Read the model definition and answer for the solid it produces. Units are mm, in the model's axes. A direction names the side the tool comes from. Coordinates: 2 decimals unless noted, no trailing zeros. Write each loop counter-clockwise with the first axis right and the second up, starting at its lowest first coordinate (ties: lowest second). Pieces come first, ordered by that corner, then holes. Notation, with made-up numbers: (5, 75) -> (21, 75) arc R18 cw to (21, 102) -> close; hole circle Ø1 at (-6.75, -40). An arc over 180 degrees is marked (long way). Answer in a Markdown table with one row per item. Add a question column.
Item 1: Section D-D on x = 11.25 is taken. Write down the section's boundary in (y, z), then the cut area to 3 significant figures.
Item 2: Section A-A on x = 18 is taken. Write down the section's boundary in (y, z).
Item 3: Given pin 1 Ø4 at (x, y) = (9.5, 38) entering from -Z; pin 2 Ø4 at (x, z) = (6, 11) entering from +Y; pin 3 Ø1 at (y, z) = (28, 55.5) entering from +X, each flat-ended and moving along its own axis, determine where each tip first touches the part or whether it passes through.
Item 4: Straight lines are drawn through the part: line 1 (Z direction, x = 3, y = 5); line 2 (Y direction, x = 22.5, z = 8); line 3 (Z direction, x = 1, y = 16). For each, find the intervals that lie inside material, in ascending order. Write a range as from..to.
Item 5: For a pull along Z with two mould halves and no side action, classify faces 6 (the face through (8.974, 32.445, 55.592)), 7 (the face through (13, 12, 0)), 8 (the face through (5, 21.55, 26)) as +Z half, -Z half, draft (parallel to the pull), parting line (faces both ways), or undercut.
Item 6: Which of the six approach directions +Z, -Z, +X, -X, +Y, -Y give full straight-line access (tool end or side, diameter ignored) to faces 1 (the face through (13, 22.05, 12)), 2 (the face through (4, 2, 26)), 3 (the face through (10, 23.55, 15)), 4 (the face through (5.86, 22.56, 50.82)), 5 (the face through (10, 44.45, 56))?
Item 7: Section B-B on z = 19 is taken. Write down the section's boundary in (x, y), then the cut area to 3 significant figures.
Item 8: Section C-C on y = 11.5 is taken. Write down the section's boundary in (x, z).
Autodesk Inventor part; units mm, degrees
ref_plane "YZ Plane" through (0, 0, 0) normal (1, 0, 0) x (0, 1, 0)
ref_plane "XZ Plane" through (0, 0, 0) normal (0, 1, 0) x (-1, 0, 0)
ref_plane "XY Plane" through (0, 0, 0) normal (0, 0, 1) x (1, 0, 0)
sketch "Sketch2" plane through (0, 0, 0) normal (1, 0, 0) x (0, 1, 0)
  line L0 (0, 0) -> (23.55, 0)
  line L1 (23.55, 0) -> (23.55, 23.55)
  line L2 (23.55, 23.55) -> (0, 23.55)
  line L3 (0, 23.55) -> (0, 0)
  line L4 (1.5, 1.5) -> (22.05, 1.5)
  line L5 (22.05, 1.5) -> (22.05, 22.05)
  line L6 (22.05, 22.05) -> (1.5, 22.05)
  line L7 (1.5, 22.05) -> (1.5, 1.5)
  dimension "d0" = 1.5
  dimension "d1" = 1.5
  dimension "d2" = 1.5
  dimension "d3" = 1.5
  dimension "d4" = 20.55
  dimension "d5" = 20.55
  dimension "widthSqAlum" = 23.55
extrude "Extrusion1" add sketch "Sketch2" along normal blind 25.4
sketch "Sketch3" plane through (0, 0, 0) normal (-1, 0, 0) x (0, 0, 1)
  line L0 (23.55, 0) -> (56.5781, 0)
  line L1 (56.5781, 0) -> (56.5781, 23.55)
  line L2 (56.5781, 23.55) -> (23.55, 23.55)
  line L3 (23.55, 23.55) -> (23.55, 0)
  dimension "d8" = 33.0281
  dimension "d9" = 23.55
extrude "Extrusion2" add sketch "Sketch3" against normal blind 2
sketch "Sketch6" plane through (0, 0, 56.5781) normal (0, 0, 1) x (1, 0, 0)
  line L0 (0, 0) -> (0, 23.55)
  line L1 (0, 0) -> (2, 0)
  line L2 (2, 23.55) -> (2, 0)
  line L3 (0, 23.55) -> (2, 23.55)
  line L4 (0, 0) -> (19.05, 0)
  line L5 (19.05, 0) -> (19.05, 44.45)
  line L6 (19.05, 44.45) -> (0, 44.45)
  line L7 (0, 44.45) -> (0, 0)
  dimension "d21" = 44.45
  dimension "d22" = 19.05
extrude "Extrusion5" add sketch "Sketch6" against normal blind 2 contours L7 L6 L5 L4 L2 L3
sketch "Sketch7" plane through (0, 44.45, 56.5781) normal (0, 0, 1) x (1, 0, 0)
  line L0 (19.05, -44.45) -> (19.05, 0)
  line L1 (19.05, 0) -> (0, 0)
  circle A0 centre (9.525, -9.525) radius 2.54
  dimension "d25" = 5.08
  dimension "d26" = 9.525
  dimension "d27" = 9.525
extrude "Extrusion6" cut sketch "Sketch7" against normal up to next
sketch "Sketch10" plane through (0, 23.55, 0) normal (0, 1, 0) x (1, 0, 0)
  line L0 (2, -23.55) -> (2, -54.5781)
  line L1 (2, -23.55) -> (25.4, -23.55)
  line L2 (0, 0) -> (0, -54.5781)
  line L3 (2, -54.5781) -> (9.62, -54.5781)
  line L4 (9.62, -54.5781) -> (2, -46.9581)
  line L5 (2, -23.55) -> (9.62, -23.55)
  line L6 (2, -31.17) -> (9.62, -23.55)
  dimension "d30" = 7.62
  dimension "d31" = 45
  dimension "d32" = 7.62
  dimension "d33" = 45
extrude "Extrusion8" add sketch "Sketch10" against normal blind 2
sketch "Sketch11" plane through (0, 0, 0) normal (0, -1, 0) x (1, 0, 0)
  line L0 (2, 23.55) -> (25.4, 23.55)
  line L1 (2, 54.5781) -> (2, 23.55)
  line L2 (19.05, 54.5781) -> (2, 54.5781)
  line L3 (2, 54.5781) -> (9.62, 54.5781)
  line L4 (9.62, 54.5781) -> (2, 46.9581)
  line L5 (2, 23.55) -> (9.62, 23.55)
  line L6 (9.62, 23.55) -> (2, 31.17)
  dimension "d44" = 45
  dimension "d45" = 45
  dimension "d46" = 7.62
  dimension "d47" = 7.62
extrude "Extrusion9" add sketch "Sketch11" against normal blind 2
equation "\"d0\" = wallThicknessSqAlum"
equation "\"d1\" = wallThicknessSqAlum"
equation "\"d2\" = wallThicknessSqAlum"
equation "\"d3\" = wallThicknessSqAlum"
equation "\"d4\" = sqAlumWidth + sqAlumTolerance"
equation "\"d5\" = sqAlumWidth + sqAlumTolerance"
equation "\"d8\" = -cameraLensHeight + screwDistanceFromFront - wallThicknessSqAlum - 0.5 * sqAlumWidth"
equation "\"d9\" = widthSqAlum"
equation "\"d21\" = heightSqAlum + d22"
equation "\"d23\" = armWallThickness"
equation "\"d26\" = 0.5 * d22"
equation "\"d27\" = 0.5 * d22"
equation "\"d28\" = armWallThickness"
equation "\"d32\" = d30"
equation "\"d33\" = d31"
equation "\"d42\" = armWallThickness"
equation "\"d44\" = d31"
equation "\"d45\" = d31"
equation "\"d46\" = d30"
equation "\"d47\" = d30"
equation "\"d48\" = armWallThickness"
equation "\"sqAlumTolerance\" = 1.5"
properties part number "cameraMount"
Results below:
| question | item | result |
|---|---|---|
| 1 | outline | (0, 0) -> (23.55, 0) -> (23.55, 23.55) -> (0, 23.55) -> close; (0, 54.58) -> (33.06, 54.58) -> (33.06, 56.58) -> (0, 56.58) -> close; (36.79, 54.58) -> (44.45, 54.58) -> (44.45, 56.58) -> (36.79, 56.58) -> close; hole (1.5, 1.5) -> (22.05, 1.5) -> (22.05, 22.05) -> (1.5, 22.05) -> close |
| 1 | area | 214 mm2 |
| 2 | outline | (0, 0) -> (23.55, 0) -> (23.55, 23.55) -> (0, 23.55) -> close; (0, 54.58) -> (44.45, 54.58) -> (44.45, 56.58) -> (0, 56.58) -> close; hole (1.5, 1.5) -> (22.05, 1.5) -> (22.05, 22.05) -> (1.5, 22.05) -> close |
| 3 | pin 1 | stops at z = 54.58 |
| 3 | pin 2 | stops at y = 23.55 |
| 3 | pin 3 | stops at x = 19.05 |
| 4 | line 1 | z = 0..1.5, 22.05..23.55, 54.58..56.58 |
| 4 | line 2 | y = 0..1.5, 22.05..23.55 |
| 4 | line 3 | z = 0..1.5, 22.05..56.58 |
| 5 | face 6 | draft |
| 5 | face 7 | -Z half |
| 5 | face 8 | undercut |
| 6 | face 1 | +X, -X |
| 6 | face 2 | +X |
| 6 | face 3 | -Z, +X, -X, +Y |
| 6 | face 4 | +X, +Y, -Y |
| 6 | face 5 | +Z, -Z, +X, -X, +Y |
| 7 | outline | (0, 0) -> (25.4, 0) -> (25.4, 1.5) -> (0, 1.5) -> close; (0, 22.05) -> (25.4, 22.05) -> (25.4, 23.55) -> (0, 23.55) -> close |
| 7 | area | 76.2 mm2 |
| 8 | outline | (0, 0) -> (25.4, 0) -> (25.4, 1.5) -> (0, 1.5) -> close; (0, 22.05) -> (25.4, 22.05) -> (25.4, 23.55) -> (2, 23.55) -> (2, 54.58) -> (19.05, 54.58) -> (19.05, 56.58) -> (0, 56.58) -> close |
